```python
from build123d import *

# Parameters (mm, degrees)
SKETCH1_R           = 5.5
BOSS_EXTRUDE1_DEPTH = 3.2
CHAMFER2_SIZE       = 1
SHELL1_T            = -1.2
SKETCH4_W           = 6.081118318
SKETCH4_H           = 6.081118318
CUT_EXTRUDE1_DEPTH  = 1.5


with BuildPart() as part:
    # Sketch1 → Boss-Extrude1 (new body)
    with BuildSketch(Plane(origin=(0, 0, 0), x_dir=(1, 0, 0), z_dir=(0, 1, 0))):
        with Locations(Location((0, 0, 0), (0, 0, 270))):
            Circle(SKETCH1_R)
    extrude(amount=BOSS_EXTRUDE1_DEPTH)

    # Chamfer2
    chamfer2_edges = [part.edges().sort_by_distance(p)[0] for p in [
        (0, 3.2, -5.5),
    ]]
    chamfer(chamfer2_edges, length=CHAMFER2_SIZE)

    # Shell1
    shell1_openings = [part.faces().sort_by_distance(p)[0] for p in [
        (0, 0, 0),
    ]]
    offset(amount=SHELL1_T, openings=shell1_openings, kind=Kind.INTERSECTION)

    # Sketch4 → Cut-Extrude1 (cut)
    with BuildSketch(Plane.XZ):
        with Locations((6.081118318, 0)):
            Rectangle(SKETCH4_W, SKETCH4_H)
    extrude(amount=-CUT_EXTRUDE1_DEPTH, mode=Mode.SUBTRACT)


solid = part.part
```
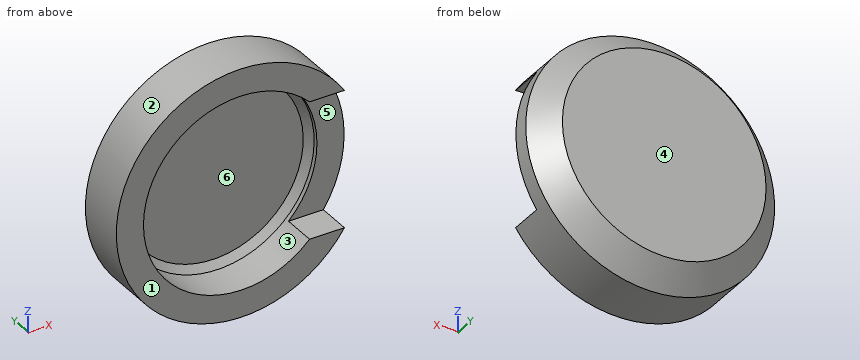
Part model, mm, in its own coordinate system. Face numbers are marked on the shaded views. A direction names the side the tool comes from. Round coordinates to 2 decimals unless told otherwise and drop trailing zeros. Loops run counter-clockwise (first coordinate to the right, second up) from the corner with the lowest first, then second, coordinate; pieces in that order, holes last.
1. Slice it at A-A (z = 0). Give the cut face in (x, y).
Solutions:
outline: (-5.5, 0) - (-4.3, 0) - (-4.3, 1.7) - (-4, 2) - (4, 2) - (4.3, 1.7) - (4.3, 1.5) - (5.5, 1.5) - (5.5, 2.2) - (4.5, 3.2) - (-4.5, 3.2) - (-5.5, 2.2) - close
2. Drill centre lines: line 1 along Z through (x, y) = (0, 0.8); line 2 along Z through (x, y) = (3, 1.3); line 3 along X through (y, z) = (0.9, 0). Where is each one in solid material? Low to high.
Solutions:
line 1: z = -5.5 to -4.3, 4.3 to 5.5
line 2: z = -4.61 to -3.08, 3.08 to 4.61
line 3: x = -5.5 to -4.3
3. Flat gauge pins, fed straight in: pin 1 (0.8 mm diameter, centred on x = 4, y = 0.5, fed in from -Z); pin 2 (1.5 mm diameter, centred on x = 4, y = 0.5, fed in from -Z); pin 3 (4 mm diameter, centred on x = -1, z = 1, fed in from -Y). Where does each tip first touch, or does it go through?
Solutions:
pin 1: stops at z = -4.16
pin 2: stops at z = -4.44
pin 3: stops at y = 2
4. 3-axis set-ups, long thin cutter, end or side, ignore diameter. For the marked faces 4, 5 and 6: which of +Z, -Z, +X, -X, +Y, -Y reach the whole face in a straight line?
Solutions:
face 4: +Z, -Z, +X, -X, +Y
face 5: +X, -Y
face 6: -Y
5. Slice it at C-C (y = 0.6). Give the cut face in (x, z).
Solutions:
outline: (3.04, -3.04) arc R4.3 cw (long way) to (3.04, 3.04) - (4.58, 3.04) arc R5.5 ccw (long way) to (4.58, -3.04) - close
6. Slice it at B-B (x = 0). Give the cut face in (y, z), and give its area (3 significant figures).
Solutions:
outline: (0, -5.5) - (2.2, -5.5) - (3.2, -4.5) - (3.2, 4.5) - (2.2, 5.5) - (0, 5.5) - (0, 4.3) - (1.7, 4.3) - (2, 4) - (2, -4) - (1.7, -4.3) - (0, -4.3) - close
area: 17.1 mm2
7. Two-plate mould, pull along Z, no slides. Class the marked faces 1, 2 and 3: pulls with the +Z half, pulls with the -Z half, needs draft (parallel to the pull), parting line crosses it, or undercut.
Solutions:
face 1: needs draft
face 2: parting line crosses it
face 3: undercut
